from build123d import *

# Parameters (mm, degrees)
F0_R     = 36.83
F1_DEPTH = 2.54
F2_R     = 38.1
F2_R_2   = 36.83
F3_DEPTH = 20.32
F4_R     = 36.83
F5_DEPTH = 2.54


with BuildPart() as f1:
    # F0 (on Right) → F1 (new body)
    with BuildSketch(Plane.YZ):
        Circle(F0_R)
    extrude(amount=-F1_DEPTH)

    # F2 (on face) → F3 (join)
    with BuildSketch(Plane.YZ):
        Circle(F2_R)
        Circle(F2_R_2, mode=Mode.SUBTRACT)
        Circle(F2_R_2)
    extrude(amount=F3_DEPTH)

    # F4 (on face) → F5 (join)
    with BuildSketch(Plane.YZ.offset(20.32)):
        Circle(F4_R)
    extrude(amount=F5_DEPTH)


solid = f1.part
Build history of the part. All positions in model axes, mm. A direction names the side the tool comes from. Round coordinates to 2 decimals unless told otherwise and drop trailing zeros. Loops run counter-clockwise (first coordinate to the right, second up) from the corner with the lowest first, then second, coordinate; pieces in that order, holes last. Notation, with made-up numbers: (22.5, -37.5) -> (62.5, -37.5) arc R17 cw to (62.5, -15.5) -> close; hole circle Ø1 at (-4, -38). An arc over 180 degrees is marked (long way). Use CSV: the item, a comma, the result in double quotes. Start each with the question number.
Q1. Saw through at A-A on z = -26. Give the cut face in (x, y), and give its area (3 significant figures).
Q2. Drill centre lines: L1, parallel to X at y = -27, z = -26; L2, parallel to Z at x = 19.75, y = 5.5; L3, parallel to Z at x = 14.5, y = -13.5. Where is each one in solid material? Low to high.
Q3. Which spindle directions (+Z, -Z, +X, -X, +Y, -Y) get a long thin tool onto all of the face, cutting with end or side? Do faces 1 (the face through (20.32, -19.9, 31.2)), 2 (the face through (0, -19.9, 31.2)), 3 (the face through (22.86, -1, 1)). Say none if no direction does.
Q4. Flat gauge pins, fed straight in: pin 1 Ø1.5 at (x, z) = (14.5, -7) entering from +Y; pin 2 Ø12 at (x, y) = (13, -4.5) entering from +Z; pin 3 Ø1.5 at (x, z) = (7, -21) entering from -Y. Where does each tip first touch, or does it go through?
Q5. Saw through at B-B on y = 10. Give the cut face in (x, z).
Q6. Saw through at C-C on x = 10.75. Give the cut face in (y, z), and give its area (3 significant figures).
Solutions:
1,outline,"(-2.54, -26.09) -> (0, -26.09) -> (0, -27.85) -> (20.32, -27.85) -> (20.32, -26.09) -> (22.86, -26.09) -> (22.86, 26.09) -> (20.32, 26.09) -> (20.32, 27.85) -> (0, 27.85) -> (0, 26.09) -> (-2.54, 26.09) -> close"
1,area,"1,400 mm^2"
2,L1,"x = 0 to 20.32"
2,L2,"z = -37.7 to 37.7"
2,L3,"z = -35.63 to 35.63"
3,face 1,"+X"
3,face 2,"-X"
3,face 3,"+Z, -Z, +X, +Y, -Y"
4,pin 1,"stops at y = 37.58"
4,pin 2,"stops at z = 38.1"
4,pin 3,"stops at y = -32.27"
5,outline,"(-2.54, -35.45) -> (0, -35.45) -> (0, -36.76) -> (20.32, -36.76) -> (20.32, -35.45) -> (22.86, -35.45) -> (22.86, 35.45) -> (20.32, 35.45) -> (20.32, 36.76) -> (0, 36.76) -> (0, 35.45) -> (-2.54, 35.45) -> close"
6,outline,"circle Ø76.2 at (0, 0)"
6,area,"4,560 mm^2"
